The model under review builds one solid part; all positions refer to its coordinate system, in mm. A direction names the side the tool comes from. Give positions to 0.01 mm unless a question says otherwise; leave off trailing zeros. Loops run counter-clockwise (first coordinate to the right, second up) from the corner with the lowest first, then second, coordinate; pieces in that order, holes last. Notation, with made-up numbers: M 12.25,69 L 56.25,69 A17 ccw 56.25,93 Z; hole C -23.75,41 d10. An arc over 180 degrees is marked long. Put each result on its own line as item: value. Start each with the question number.
from build123d import *

# Parameters (mm, degrees)
SKETCH_1_W          = 60
SKETCH_1_H          = 20
EXTRUDE_1_DEPTH     = 1.2
CUT_EXTRUDE_1_REACH = 33.646
SKETCH_4_R          = 3.25
SKETCH_4_W          = 9.6
SKETCH_4_H          = 3.4
SKETCH_4_W_2        = 7
SKETCH_4_H_2        = 3.5
SKETCH_4_W_3        = 8
SKETCH_4_H_3        = 2.9
SKETCH_4_W_4        = 8.4
SKETCH_4_H_4        = 3.2
SKETCH_4_W_5        = 6.5
FILLET_2_R          = 1
CHAMFER_1_SIZE      = 0.6
SKETCH_5_W          = 1.5
SKETCH_5_H          = 8
EXTRUDE_2_DEPTH     = 1.2
SKETCH_6_W          = 28.5
SKETCH_6_H          = 1.6
EXTRUDE_3_DEPTH     = 4
FILLET_3_R          = 1
CHAMFER_2_SIZE      = 1
CHAMFER_4_SIZE      = 1
SKETCH_7_W          = 2
SKETCH_7_H          = 20
CUT_EXTRUDE_2_DEPTH = 5
EXTRUDE_5_DEPTH     = 1.2
FILLET_5_R          = 2
FILLET_6_R          = 0.5
CHAMFER_5_SIZE      = 2
CHAMFER_5_SIZE_2    = 2.383507185
CHAMFER_6_SIZE      = 2
CHAMFER_6_SIZE_2    = 2.383507185


with BuildPart() as part:
    # 草图1 → 凸台-拉伸1 (new body)
    with BuildSketch(Plane(origin=(0, 0, 0), x_dir=(1, 0, 0), z_dir=(0, 1, 0))):
        Rectangle(SKETCH_1_W, SKETCH_1_H)
    extrude(amount=EXTRUDE_1_DEPTH)

    # 草图4 → 切除-拉伸1 (cut, up to next)
    with BuildSketch(Plane(origin=(0, 1.2, 0), x_dir=(1, 0, 0), z_dir=(0, 1, 0)), mode=Mode.PRIVATE) as cut_extrude_1_sk1:
        with Locations(Location((22.298485985, 5.48318929, 0), (0, 0, 270))):
            Circle(SKETCH_4_R)
    cut_extrude_1_tool1 = extrude(cut_extrude_1_sk1.sketch, amount=-CUT_EXTRUDE_1_REACH, mode=Mode.PRIVATE) & part.part
    # 草图4 → 切除-拉伸1 (cut, up to next)
    with BuildSketch(Plane(origin=(0, 1.2, 0), x_dir=(1, 0, 0), z_dir=(0, 1, 0)), mode=Mode.PRIVATE) as cut_extrude_1_sk2:
        with Locations((-20.471722325, 4.1)):
            Rectangle(SKETCH_4_W, SKETCH_4_H)
    cut_extrude_1_tool2 = extrude(cut_extrude_1_sk2.sketch, amount=-CUT_EXTRUDE_1_REACH, mode=Mode.PRIVATE) & part.part
    # 草图4 → 切除-拉伸1 (cut, up to next)
    with BuildSketch(Plane(origin=(0, 1.2, 0), x_dir=(1, 0, 0), z_dir=(0, 1, 0)), mode=Mode.PRIVATE) as cut_extrude_1_sk3:
        with Locations((-5.682926277, 4.05)):
            Rectangle(SKETCH_4_W_2, SKETCH_4_H_2)
    cut_extrude_1_tool3 = extrude(cut_extrude_1_sk3.sketch, amount=-CUT_EXTRUDE_1_REACH, mode=Mode.PRIVATE) & part.part
    # 草图4 → 切除-拉伸1 (cut, up to next)
    with BuildSketch(Plane(origin=(0, 1.2, 0), x_dir=(1, 0, 0), z_dir=(0, 1, 0)), mode=Mode.PRIVATE) as cut_extrude_1_sk4:
        with Locations((7.788485985, 4.05)):
            Rectangle(SKETCH_4_W_2, SKETCH_4_H_2)
    cut_extrude_1_tool4 = extrude(cut_extrude_1_sk4.sketch, amount=-CUT_EXTRUDE_1_REACH, mode=Mode.PRIVATE) & part.part
    # 草图4 → 切除-拉伸1 (cut, up to next)
    with BuildSketch(Plane(origin=(0, 1.2, 0), x_dir=(1, 0, 0), z_dir=(0, 1, 0)), mode=Mode.PRIVATE) as cut_extrude_1_sk5:
        with Locations((21.05, -3.084803861)):
            Rectangle(SKETCH_4_W_3, SKETCH_4_H_3)
    cut_extrude_1_tool5 = extrude(cut_extrude_1_sk5.sketch, amount=-CUT_EXTRUDE_1_REACH, mode=Mode.PRIVATE) & part.part
    # 草图4 → 切除-拉伸1 (cut, up to next)
    with BuildSketch(Plane(origin=(0, 1.2, 0), x_dir=(1, 0, 0), z_dir=(0, 1, 0)), mode=Mode.PRIVATE) as cut_extrude_1_sk6:
        with Locations((7.4, -3.234803861)):
            Rectangle(SKETCH_4_W_4, SKETCH_4_H_4)
    cut_extrude_1_tool6 = extrude(cut_extrude_1_sk6.sketch, amount=-CUT_EXTRUDE_1_REACH, mode=Mode.PRIVATE) & part.part
    # 草图4 → 切除-拉伸1 (cut, up to next)
    with BuildSketch(Plane(origin=(0, 1.2, 0), x_dir=(1, 0, 0), z_dir=(0, 1, 0)), mode=Mode.PRIVATE) as cut_extrude_1_sk7:
        with Locations((-7.25, -3.384803861)):
            Rectangle(SKETCH_4_W_5, SKETCH_4_H_2)
    cut_extrude_1_tool7 = extrude(cut_extrude_1_sk7.sketch, amount=-CUT_EXTRUDE_1_REACH, mode=Mode.PRIVATE) & part.part
    # 草图4 → 切除-拉伸1 (cut, up to next)
    with BuildSketch(Plane(origin=(0, 1.2, 0), x_dir=(1, 0, 0), z_dir=(0, 1, 0)), mode=Mode.PRIVATE) as cut_extrude_1_sk8:
        with Locations((-20.471722325, -3.334803861)):
            Rectangle(SKETCH_4_W, SKETCH_4_H)
    cut_extrude_1_tool8 = extrude(cut_extrude_1_sk8.sketch, amount=-CUT_EXTRUDE_1_REACH, mode=Mode.PRIVATE) & part.part
    add(cut_extrude_1_tool1.solids().sort_by_distance((22.298486, 1.2, -5.483189))[0], mode=Mode.SUBTRACT)
    add(cut_extrude_1_tool2.solids().sort_by_distance((-20.471722, 1.2, -4.1))[0], mode=Mode.SUBTRACT)
    add(cut_extrude_1_tool3.solids().sort_by_distance((-5.682926, 1.2, -4.05))[0], mode=Mode.SUBTRACT)
    add(cut_extrude_1_tool4.solids().sort_by_distance((7.788486, 1.2, -4.05))[0], mode=Mode.SUBTRACT)
    add(cut_extrude_1_tool5.solids().sort_by_distance((21.05, 1.2, 3.084804))[0], mode=Mode.SUBTRACT)
    add(cut_extrude_1_tool6.solids().sort_by_distance((7.4, 1.2, 3.234804))[0], mode=Mode.SUBTRACT)
    add(cut_extrude_1_tool7.solids().sort_by_distance((-7.25, 1.2, 3.384804))[0], mode=Mode.SUBTRACT)
    add(cut_extrude_1_tool8.solids().sort_by_distance((-20.471722, 1.2, 3.334804))[0], mode=Mode.SUBTRACT)

    # 圆角2
    fillet_2_edges = [part.edges().sort_by_distance(p)[0] for p in [
        (-9.182926277, 0.6, -5.8),
        (-2.182926277, 0.6, -5.8),
        (4.288485985, 0.6, -5.8),
        (11.288485985, 0.6, -5.8),
        (17.05, 0.6, 4.534803861),
        (25.05, 0.6, 4.534803861),
        (3.2, 0.6, 4.834803861),
        (3.2, 0.6, 1.634803861),
        (11.6, 0.6, 1.634803861),
        (11.6, 0.6, 4.834803861),
        (-10.5, 0.6, 5.134803861),
        (-10.5, 0.6, 1.634803861),
        (-4, 0.6, 1.634803861),
        (-4, 0.6, 5.134803861),
        (-25.271722325, 0.6, 5.034803861),
        (-25.271722325, 0.6, 1.634803861),
        (-15.671722325, 0.6, 1.634803861),
        (-15.671722325, 0.6, 5.034803861),
        (-25.271722325, 0.6, -2.4),
        (-25.271722325, 0.6, -5.8),
        (-15.671722325, 0.6, -5.8),
        (-15.671722325, 0.6, -2.4),
    ]]
    fillet(fillet_2_edges, radius=FILLET_2_R)

    # 倒角1
    chamfer_1_edges = [part.edges().sort_by_distance(p)[0] for p in [
        (-9.182926277, 0.6, -2.3),
        (-2.182926277, 0.6, -2.3),
        (4.288485985, 0.6, -2.3),
        (11.288485985, 0.6, -2.3),
        (17.05, 0.6, 1.634803861),
        (25.05, 0.6, 1.634803861),
    ]]
    chamfer(chamfer_1_edges, length=CHAMFER_1_SIZE)

    # 草图5 → 凸台-拉伸2 (add)
    with BuildSketch(Plane.XZ):
        with Locations((-13.15891381, -0.88318929)):
            Rectangle(SKETCH_5_W, SKETCH_5_H)
        with Locations((13.84108619, -0.88318929)):
            Rectangle(SKETCH_5_W, SKETCH_5_H)
    extrude(amount=EXTRUDE_2_DEPTH)

    # 草图6 → 凸台-拉伸3 (add)
    with BuildSketch(Plane.XZ):
        with Locations((0.34108619, -0.2)):
            Rectangle(SKETCH_6_W, SKETCH_6_H)
    extrude(amount=EXTRUDE_3_DEPTH)

    # 圆角3
    fillet_3_edges = [part.edges().sort_by_distance(p)[0] for p in [
        (-13.90891381, -4, -0.2),
        (14.59108619, -4, -0.2),
    ]]
    fillet(fillet_3_edges, radius=FILLET_3_R)

    # 倒角2
    chamfer_2_edges = [part.edges().sort_by_distance(p)[0] for p in [
        (-13.15891381, -1.2, -4.88318929),
        (-13.15891381, -1.2, 3.11681071),
        (13.84108619, -1.2, -4.88318929),
        (13.84108619, -1.2, 3.11681071),
    ]]
    chamfer(chamfer_2_edges, length=CHAMFER_2_SIZE)

    # 倒角4
    chamfer_4_edges = [part.edges().sort_by_distance(p)[0] for p in [
        (-5.682926277, 0, -5.8),
        (-2.182926277, 0, -3.85),
        (7.788485985, 0, -5.8),
        (11.288485985, 0, -3.85),
        (21.05, 0, 4.534803861),
        (17.05, 0, 2.884803861),
        (-2.475819496, 0, -5.507106781),
        (-8.890033058, 0, -5.507106781),
        (4.581379204, 0, -5.507106781),
        (10.995592766, 0, -5.507106781),
        (24.757106781, 0, 4.241910642),
        (17.342893219, 0, 4.241910642),
        (-5.682926277, 0, -2.3),
        (-9.182926277, 0, -3.85),
        (7.788485985, 0, -2.3),
        (4.288485985, 0, -3.85),
        (21.05, 0, 1.634803861),
        (25.05, 0, 2.884803861),
        (-8.882926277, 0, -2.6),
        (-2.482926277, 0, -2.6),
        (4.588485985, 0, -2.6),
        (10.988485985, 0, -2.6),
        (17.35, 0, 1.934803861),
        (24.75, 0, 1.934803861),
    ]]
    chamfer(chamfer_4_edges, length=CHAMFER_4_SIZE)

    # 草图7 → 切除-拉伸2 (cut)
    with BuildSketch(Plane(origin=(0, 1.2, 0), x_dir=(1, 0, 0), z_dir=(0, 1, 0))):
        with Locations((29, 0)):
            Rectangle(SKETCH_7_W, SKETCH_7_H)
        with Locations((-29, 0)):
            Rectangle(SKETCH_7_W, SKETCH_7_H)
    extrude(amount=-CUT_EXTRUDE_2_DEPTH, mode=Mode.SUBTRACT)

    # 草图11 → 凸台-拉伸5 (add)
    with BuildSketch(Plane(origin=(0, 1.2, 0), x_dir=(1, 0, 0), z_dir=(0, 1, 0))):
        Polygon((28, 10), (30.2, 10), (30.2, 2), (31.7, 2), (31.7, 0), (28.7, 0), (28.7, 7), (28, 7), align=None)
        Polygon((-28, 10), (-30.2, 10), (-30.2, 2), (-31.7, 2), (-31.7, 0), (-28.7, 0), (-28.7, 7), (-28, 7), align=None)
    extrude(amount=-EXTRUDE_5_DEPTH)

    # 圆角5
    fillet_5_edges = [part.edges().sort_by_distance(p)[0] for p in [
        (28, 0.6, 10),
        (-28, 0.6, 10),
        (30.2, 0.6, -10),
        (-30.2, 0.6, -10),
    ]]
    fillet(fillet_5_edges, radius=FILLET_5_R)

    # 圆角6
    # the kernel refuses this fillet: 0.5 mm, written as the material it adds along each edge
    with BuildSketch(Plane(origin=(28, 1.2, -7), x_dir=(0, 0, 1), z_dir=(0, -1, 0)), Plane(origin=(28.7, 1.2, -7), x_dir=(-1, 0, 0), z_dir=(0, -1, 0))) as fillet_6_piece_1:
        with BuildLine():
            CenterArc((FILLET_6_R, -FILLET_6_R), FILLET_6_R, 90, 90)
            Line((0, -FILLET_6_R), (0, 0))
            Line((0, 0), (FILLET_6_R, 0))
        make_face()
    extrude(amount=1.2)
    with BuildSketch(Plane(origin=(-28, 1.2, -7), x_dir=(0, 0, 1), z_dir=(0, -1, 0)), Plane(origin=(-28.7, 1.2, -7), x_dir=(1, 0, 0), z_dir=(0, -1, 0))) as fillet_6_piece_2:
        with BuildLine():
            CenterArc((FILLET_6_R, FILLET_6_R), FILLET_6_R, 180, 90)
            Line((0, FILLET_6_R), (0, 0))
            Line((0, 0), (FILLET_6_R, 0))
        make_face()
    extrude(amount=1.2)

    # 倒角5
    # the kernel refuses this chamfer: 2.383507185, 2 mm, written as the material it takes off along each edge
    with BuildSketch(Plane(origin=(31.7, 7.343265966, 0), x_dir=(-0.9993728857116148, 0, 0.03540953691366325), z_dir=(0, -1, 0))) as chamfer_5_piece_1:
        Polygon((CHAMFER_5_SIZE * 0.999372885712, CHAMFER_5_SIZE * 0.0354095369137), (-CHAMFER_5_SIZE_2 * 0.0354095369165, CHAMFER_5_SIZE_2 * 0.999372885791), (0, 0), align=None)
    extrude(amount=13.486531933, mode=Mode.SUBTRACT)

    # 倒角6
    # the kernel refuses this chamfer: 2.383507185, 2 mm, written as the material it takes off along each edge
    with BuildSketch(Plane(origin=(-31.7, 7.343265966, 0), x_dir=(0.9993728857116148, 0, 0.03540953691366311), z_dir=(0, -1, 0))) as chamfer_6_piece_1:
        Polygon((CHAMFER_6_SIZE * 0.999372885712, -CHAMFER_6_SIZE * 0.0354095369137), (-CHAMFER_6_SIZE_2 * 0.0354095369165, -CHAMFER_6_SIZE_2 * 0.999372885791), (0, 0), align=None)
    extrude(amount=13.486531933, mode=Mode.SUBTRACT)


solid = part.part
(1) Draft analysis for pull direction X (two halves, no side actions). For faces 6 (the flat face through (13.091, -1, 2)), 7 (the flat face through (0, 1, -10)), 8 (the cylindrical face through (27.4, 0.59, 9.43)), state which applies: +X half, -X half, draft (parallel to the pull), parting line (faces both ways), or undercut.
(2) To check wall thickness, follow L1, parallel to X at y = 0.2, z = -6.75; L2, parallel to Y at x = -4.5, z = 8; L3, parallel to Z at x = -5.5, y = 0.25. State the ranges of each line that lie inside material, in increasing order. Write a range as [from, to].
(3) We need section B-B, the plane y = -2.15. Write out the cut boundary in (x, z).
(4) Insertion check: pin 1 (2 mm diameter, centred on x = -2.5, y = -1.5, fed in from +Z); pin 2 (0.6 mm diameter, centred on y = 1, z = 3, fed in from -X); pin 3 (2 mm diameter, centred on x = 22.5, y = -2.5, fed in from -Z); pin 4 (12 mm diameter, centred on x = -22, z = 2, fed in from -Y). Each pin has a flat end and moves straight along its axis. Give the tip position at first contact, or say it passes through.
(5) We need section C-C, the plane z = 6.75. Write out the cut boundary in (x, y).
(6) We need section A-A, the plane x = -21. Write out the cut boundary in (y, z).
(7) For faces 1 (the flat face through (14.591, -1, -1)), 2 (the flat face through (3.8, 0.51, -3.66)), 3 (the flat face through (-13.169, -0.693, -4.39)), 4 (the flat face through (30.53, 0.61, -0.99)), 5 (the flat face through (7, 1, 1.635)), list the 3-axis set-ups (+Z, -Z, +X, -X, +Y, -Y) from which the entire face can be reached by the end or side of a thin tool; tool diameter is ignored.
Check sheet entries:
1. face 6: undercut
1. face 7: draft
1. face 8: +X half
2. L1: x = [-30.2, -28.63], [-28.07, 19.31], [25.29, 28.07], [28.63, 30.2]
2. L2: y = [0, 1.2]
2. L3: z = [-10, -6.55], [-1.55, 1.63], [5.13, 10]
3. outline: M -13.91,-1 L 14.59,-1 L 14.59,0.6 L -13.91,0.6 Z
4. pin 1: stops at z = 0.6
4. pin 2: stops at x = -28
4. pin 3: passes through
4. pin 4: stops at y = 0
5. outline: M -28,0 L 28,0 L 28,1.2 L -28,1.2 Z
6. outline: M 0,-10 L 1.2,-10 L 1.2,-5.8 L 0,-5.8 Z; M 0,-2.4 L 1.2,-2.4 L 1.2,1.63 L 0,1.63 Z; M 0,5.03 L 1.2,5.03 L 1.2,10 L 0,10 Z
7. face 1: +Z, -Z, +X, -Y
7. face 2: -Y
7. face 3: -Z, +X, -X, -Y
7. face 4: +Z, +X, +Y, -Y
7. face 5: +Y, -Y
